The model under review builds one solid part; all positions refer to its coordinate system, in mm. Round coordinates to 2 decimals unless told otherwise and drop trailing zeros. Loops run counter-clockwise (first coordinate to the right, second up) from the corner with the lowest first, then second, coordinate; pieces in that order, holes last. Notation, with made-up numbers: (61.5, -36.75) -> (94.5, -36.75) arc R5 cw to (94.5, -31.75) -> close; hole circle Ø1 at (19.25, 3.25). An arc over 180 degrees is marked (long way). Use CSV: the item, a comma, the result in double quotes. Start each with the question number.
```python
from build123d import *

# Parameters (mm, degrees)
F_3_8_0_3750_DOWEL_HOLE1_D = 9.525
FILLET2_R                  = 1.5875
CHAMFER3_SIZE              = 1.42875


with BuildPart() as part:
    # Sketch1 → Revolve1 (revolve)
    with BuildSketch(Plane.XY):
        Polygon((0, 0), (0, 9.525), (25.4, 9.525), (25.4, 4.7625), (63.5, 4.7625), (63.5, 0), align=None)
    revolve(axis=Axis((0, 0, 0), (1, 0, 0)))

    # 3/8 (0.3750) Dowel Hole1 (through all)
    with Locations(Plane.XY.offset(9.525)):
        with Locations((9.525, 0)):
            Hole(F_3_8_0_3750_DOWEL_HOLE1_D / 2)

    # Fillet2
    fillet2_edges = [part.edges().sort_by_distance(p)[0] for p in [
        (0, -9.525, 0),
    ]]
    fillet(fillet2_edges, radius=FILLET2_R)

    # Chamfer3
    chamfer3_edges = [part.edges().sort_by_distance(p)[0] for p in [
        (63.5, -4.7625, 0),
    ]]
    chamfer(chamfer3_edges, length=CHAMFER3_SIZE)


solid = part.part
```
1. For line 1 along X through (y, z) = (0, -2.5); line 2 along X through (y, z) = (0, 5.5); line 3 along X through (y, z) = (-5.25, 6), list the stretches that pass through material, from the lowest coordinate up. Write a range as from..to.
2. The part is to be moulded in two halves that separate along X. For faces 1 (the face through (43.99, -3.78, -2.9)), 2 (the face through (0, 0, 0)), 3 (the face through (6.965, 4.016, -0.133)), 4 (the face through (25.4, -2.3, 4.4)), say which applies: pulls with the +X half, pulls with the -X half, needs draft (parallel to the pull), parting line crosses it, or undercut.
3. Take a section at D-D, the plane x = 21.5. Give the boundary of the cut face in (y, z) (3 decimals).
4. Take a section at A-A, the plane y = 0. Give the boundary of the cut face in (x, z) (1 decimal).
5. Take a section at B-B, the plane z = 0. Give the boundary of the cut face in (x, y) (1 decimal), then the cut area to 3 significant figures.
6. Take a section at C-C, the plane x = 11. Give the boundary of the cut face in (y, z) (3 decimals), then the cut area to 3 significant figures.
7. Clearance check with flat-ended pins moving along their axes: P1, Ø5, axis at x = 20, y = -3.5, coming from the +Z side; P2, Ø2, axis at x = 39, y = -4.5, coming from the -Z side; P3, Ø1, axis at x = 22.5, y = 6, coming from the -Z side. State where each tip first meets the part, or that it passes through.
Results:
1,line 1,"0..4.76, 14.29..63.5"
1,line 2,"0..4.76, 14.29..25.4"
1,line 3,"0..25.4"
2,face 1,"needs draft"
2,face 2,"pulls with the -X half"
2,face 3,"undercut"
2,face 4,"pulls with the +X half"
3,outline,"circle Ø19.05 at (0, 0)"
4,outline,"(0, -7.9) arc R1.6 ccw to (1.6, -9.5) -> (4.8, -9.5) -> (4.8, 9.5) -> (1.6, 9.5) arc R1.6 ccw to (0, 7.9) -> close; (14.3, -9.5) -> (25.4, -9.5) -> (25.4, -4.8) -> (62.1, -4.8) -> (63.5, -3.3) -> (63.5, 3.3) -> (62.1, 4.8) -> (25.4, 4.8) -> (25.4, 9.5) -> (14.3, 9.5) -> close"
5,outline,"(0, -7.9) arc R1.6 ccw to (1.6, -9.5) -> (25.4, -9.5) -> (25.4, -4.8) -> (62.1, -4.8) -> (63.5, -3.3) -> (63.5, 3.3) -> (62.1, 4.8) -> (25.4, 4.8) -> (25.4, 9.5) -> (1.6, 9.5) arc R1.6 ccw to (0, 7.9) -> close; hole circle Ø9.5 at (9.5, 0)"
5,area,"772 mm²"
6,outline,"(-4.528, -8.38) -> (-4.528, 8.38) arc R9.525 ccw to start; (4.528, -8.38) arc R9.525 ccw to (4.528, 8.38) -> close"
6,area,"119 mm²"
7,P1,"z = 9.47"
7,P2,"z = -3.23"
7,P3,"z = -7.78"
